Can you work these out from the model? Positions are in its coordinate system, mm. Give positions to 0.01 mm unless a question says otherwise; leave off trailing zeros. Order: outer loops, then holes, each group sorted by start corner. A loop starts at its lowest first (then second) coordinate and runs counter-clockwise, first axis right, second up. Notation, with made-up numbers: (16, 37.25) - (68, 37.25) arc R30 cw to (68, 73.25) - close; hole circle Ø3 at (39.5, 7.5). An arc over 180 degrees is marked (long way). Return JSON: item names as keys, results as strings.
```python
from build123d import *

# Parameters (mm, degrees)
BOSS_EXTRUDE1_DEPTH         = 6
TAP_DRILL_FOR_M8X1_0_TAP2_D = 7


with BuildPart() as part:
    # Sketch1 → Boss-Extrude1 (new body)
    with BuildSketch(Plane(origin=(0, 0, 0), x_dir=(0, 0, -1), z_dir=(1, 0, 0))):
        Polygon((-28.922954929, 86.159638097), (-28.922954929, 94.159638097), (2.104632598, 76.455689895), (5.358525743, 83.764053556), (26.502792929, 54.9706353), (32.447951533, 60.323680151), (40.052862492, 25.419435438), (47.661314622, 27.891571393), (40.411911161, -7.088238772), (48.368086324, -7.924466478), (27.517856159, -36.931515135), (34.44605939, -40.931515135), (3.600196736, -58.95022005), (8.302478754, -65.422356005), (-27.20548651, -69.337119405), (-25.542192984, -77.162300211), (-59.572611085, -66.296223938), (-61.235904612, -74.121404744), (-87.904607103, -50.353332102), (-92.606889121, -56.825468057), (-107.302615065, -24.265114732), (-114.230818295, -28.265114732), (-114.412543169, 7.457538386), (-122.368718332, 6.62131068), (-108.005020253, 39.329492336), (-115.613472384, 41.801628291), (-89.187965242, 65.839796731), (-95.133123845, 71.192841582), (-61.215017893, 82.404579105), (-64.468911037, 89.712942766), align=None)
    extrude(amount=BOSS_EXTRUDE1_DEPTH)

    # Tap Drill for M8x1.0 Tap2 (through all)
    with Locations(Plane.ZY):
        with Locations((36.235904612, 8.321002744)):
            Hole(TAP_DRILL_FOR_M8X1_0_TAP2_D / 2)


solid = part.part
```
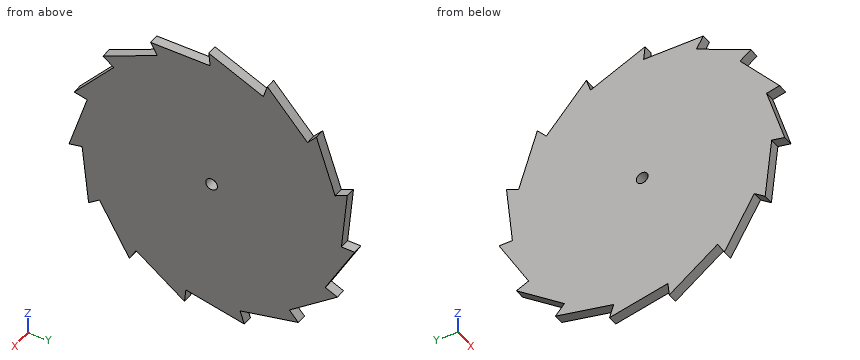
1. Suppose I cut it at C-C (z = -22). List the corners of the cut face in (x, y) for me, plus the area to 3 significant figures.
Checks:
{"outline": "(0, -48.2) - (6, -48.2) - (6, 61.1) - (0, 61.1) - close", "area": "656 mm^2"}
2. If I drill on L1, parallel to Z at x = 2.7, y = -54; L2, parallel to Y at x = 5.65, z = 110.5; L3, parallel to Z at x = 1.1, y = 83.5, over which ranges is the centre line in solid material (lowest first)? Write a range as [from, to].
Checks:
{"L1": "[-12.07, 83.81], [90.55, 93.88]", "L2": "[-26.11, 33.65], [40.14, 46.45]", "L3": "[-5.55, -5.24], [10.24, 61.7]"}
3. Suppose I cut it at B-B (y = 51). List the corners of the cut face in (x, z) for me, plus the area to 3 significant figures.
Checks:
{"outline": "(0, -34.48) - (6, -34.48) - (6, 105.5) - (0, 105.5) - close", "area": "840 mm^2"}
4. For pin 1 Ø2 at (x, z) = (5, 95) entering from -Y, with a flat end and sliding along its axis, tell me the tip position at first contact or that it passes through.
Checks:
{"pin 1": "y = -53.74"}
